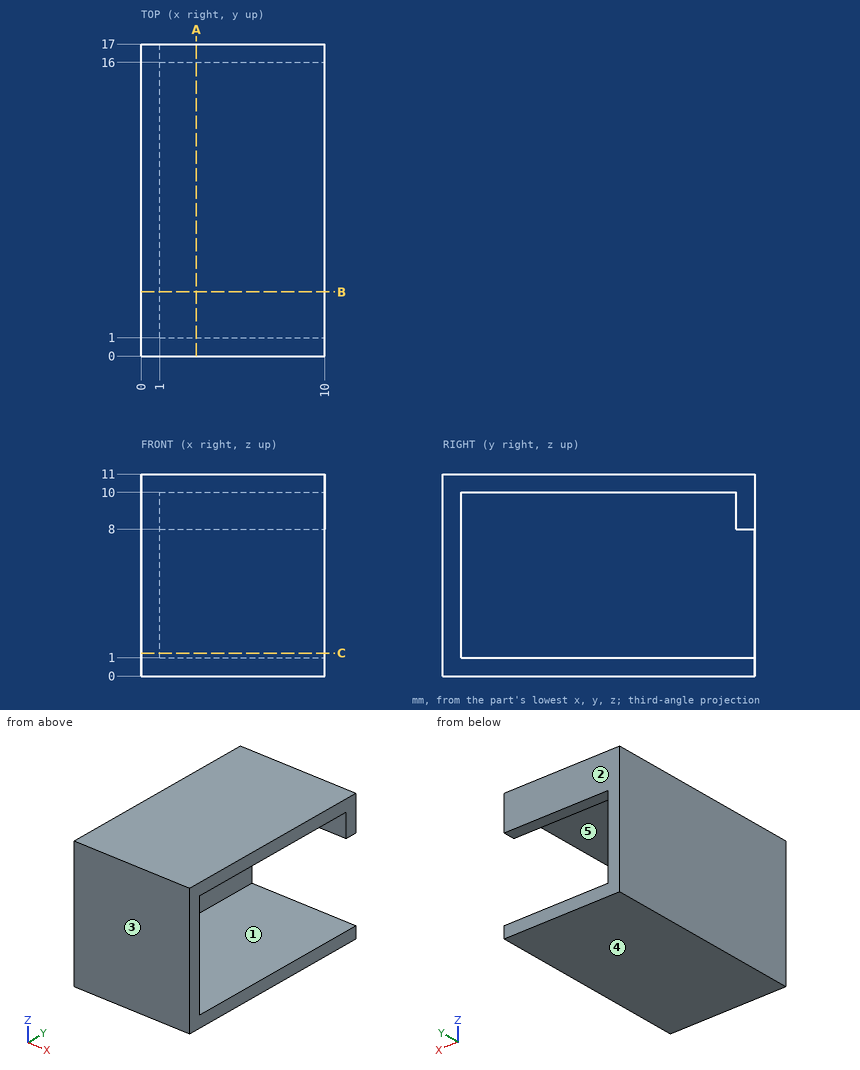
Check sheet for the drawn part. Datum: minimum x, y, z corner. Units: mm. A direction names the side the tool comes from. Give positions to 0.01 mm unless a question says otherwise; leave off trailing zeros. Order: outer loops, then holes, each group sorted by start corner. A loop starts at its lowest first (then second) coordinate and runs counter-clockwise, first axis right, second up.
1. Sectioned sample at A-A (x = 3). Record the boundary of the cut face in (y, z).
Completed:
outline: (0, 0) - (17, 0) - (17, 1) - (1, 1) - (1, 10) - (16, 10) - (16, 8) - (17, 8) - (17, 11) - (0, 11) - close
2. Draft check along Y on the marked faces 3, 4 and 5. Enter one of: pulls with the +Y half, pulls with the -Y half, needs draft (parallel to the pull), parting line crosses it, or undercut.
Completed:
face 3: pulls with the -Y half
face 4: needs draft
face 5: undercut
3. Depth check by flat-ended pin: pin 1 (0.5 mm diameter, centred on x = 4.5, y = 16.5, fed in from -Z); pin 2 (4.5 mm diameter, centred on x = 5, z = 4, fed in from +Y); pin 3 (4.5 mm diameter, centred on y = 11.5, z = 5, fed in from +X). Enter the tip coordinate at first touch or a pass-through.
Completed:
pin 1: stops at z = 0
pin 2: stops at y = 1
pin 3: stops at x = 1
4. Sectioned sample at C-C (z = 1.25). Record the boundary of the cut face in (x, y).
Completed:
outline: (0, 0) - (10, 0) - (10, 1) - (1, 1) - (1, 17) - (0, 17) - close
5. Scan lines: line 1 (Z direction, x = 3.75, y = 5.5); line 2 (Y direction, x = 3.5, z = 9.25); line 3 (X direction, y = 7.75, z = 8). Record each from-to range of solid material in increasing order.
Completed:
line 1: z = 0 to 1, 10 to 11
line 2: y = 0 to 1, 16 to 17
line 3: x = 0 to 1
6. Sectioned sample at B-B (y = 3.5). Record the boundary of the cut face in (x, z).
Completed:
outline: (0, 0) - (10, 0) - (10, 1) - (1, 1) - (1, 10) - (10, 10) - (10, 11) - (0, 11) - close
7. Access from +Z, -Z, +X, -X, +Y, -Y to the whole of each face (thin tool, end or side, straight path). Record for the marked faces 1 and 2.
Completed:
face 1: +X, +Y
face 2: +Z, -Z, +X, -X, +Y
